```python
from build123d import *

# Parameters (mm, degrees)
EXTRUDE_1_DEPTH = 1


with BuildPart() as part:
    # 草图1 → 凸台-拉伸1 (new body)
    with BuildSketch(Plane.XY):
        Polygon((-75, -66.463368351), (-75, -65.063368351), (75, -65.063368351), (75, -62.463368351), (-75, -62.463368351), (-75, -61.063368351), (75, -61.063368351), (75, -58.463368351), (-75, -58.463368351), (-75, -57.063368351), (75, -57.063368351), (75, -54.463368351), (-75, -54.463368351), (-75, -53.063368351), (75, -53.063368351), (75, -50.463368351), (-75, -50.463368351), (-75, -49.063368351), (75, -49.063368351), (75, -46.463368351), (-75, -46.463368351), (-75, -45.063368351), (75, -45.063368351), (75, -42.463368351), (-75, -42.463368351), (-75, -41.063368351), (75, -41.063368351), (75, -38.463368351), (-75, -38.463368351), (-75, -37.063368351), (75, -37.063368351), (75, -34.463368351), (-75, -34.463368351), (-75, -33.063368351), (75, -33.063368351), (75, -30.463368351), (-75, -30.463368351), (-75, -29.063368351), (75, -29.063368351), (75, -26.463368351), (-75, -26.463368351), (-75, -25.063368351), (75, -25.063368351), (75, -22.463368351), (-75, -22.463368351), (-75, -21.063368351), (75, -21.063368351), (75, -18.463368351), (-75, -18.463368351), (-75, -17.063368351), (75, -17.063368351), (75, -14.463368351), (-75, -14.463368351), (-75, -13.063368351), (75, -13.063368351), (75, -10.463368351), (-75, -10.463368351), (-75, -9.063368351), (75, -9.063368351), (75, -6.463368351), (-75, -6.463368351), (-75, -5.063368351), (75, -5.063368351), (75, -2.463368351), (-75, -2.463368351), (-75, -1.063368351), (75, -1.063368351), (75, 1.536631649), (-75, 1.536631649), (-75, 2.936631649), (75, 2.936631649), (75, 5.536631649), (-75, 5.536631649), (-75, 6.936631649), (75, 6.936631649), (75, 9.536631649), (-75, 9.536631649), (-75, 10.936631649), (75, 10.936631649), (75, 13.536631649), (-75, 13.536631649), (-75, 14.936631649), (75, 14.936631649), (75, 17.536631649), (-75, 17.536631649), (-75, 18.936631649), (75, 18.936631649), (75, 21.536631649), (-75, 21.536631649), (-75, 22.936631649), (75, 22.936631649), (75, 25.536631649), (-75, 25.536631649), (-75, 26.936631649), (75, 26.936631649), (75, 29.536631649), (-75, 29.536631649), (-75, 30.936631649), (75, 30.936631649), (75, 33.536631649), (-75, 33.536631649), (-75, 34.936631649), (75, 34.936631649), (75, 37.536631649), (-75, 37.536631649), (-75, 38.936631649), (75, 38.936631649), (75, 41.536631649), (-75, 41.536631649), (-75, 42.936631649), (75, 42.936631649), (75, 45.536631649), (-75, 45.536631649), (-75, 46.936631649), (75, 46.936631649), (75, 49.536631649), (-75, 49.536631649), (-75, 50.936631649), (75, 50.936631649), (75, 53.536631649), (-75, 53.536631649), (-75, 54.936631649), (75, 54.936631649), (75, 57.536631649), (-75, 57.536631649), (-75, 58.936631649), (75, 58.936631649), (75, 61.536631649), (-75, 61.536631649), (-75, 62.936631649), (75, 62.936631649), (75, 65.536631649), (-75, 65.536631649), (-75, 66.936631649), (75, 66.936631649), (75, 69.536631649), (-75, 69.536631649), (-75, 70.936631649), (75, 70.936631649), (75, 80.236631649), (-85, 80.236631649), (-85, -79.763368351), (75, -79.763368351), (75, -70.463368351), (-75, -70.463368351), (-75, -69.063368351), (75, -69.063368351), (75, -66.463368351), align=None)
    extrude(amount=EXTRUDE_1_DEPTH)


solid = part.part
```
Source: CAD feature listing. Evaluate the final solid. Frame: model axes, mm. Round coordinates to 2 decimals unless told otherwise and drop trailing zeros.
1. Contact query for flat-ended pins moving along their axis: pin 1 (0.5 mm diameter, centred on y = 26.5, z = 0.5, fed in from +X); pin 2 (2 mm diameter, centred on x = -51.5, y = 39.5, fed in from -Z). Output: stop coordinate, or through.
2. Ray query, L1, parallel to X at y = -1.5, z = 0.25. Return the intervals inside material, ascending.
3. Section query A-A on x = -34. Give the number of separate pieces and of enclosed holes in the cut face, and give its area (3 significant figures).
Answers below:
1. pin 1: stops at x = -75
1. pin 2: stops at z = 0
2. L1: x = -85 to -75
3. separate pieces: 37
3. enclosed holes: 0
3. area: 110 mm2
